Geometry: see drawing. Coordinates: mm, zero at the bounding-box minimum. Coordinates: 2 decimals unless noted, no trailing zeros. Write each loop counter-clockwise with the first axis right and the second up, starting at its lowest first coordinate (ties: lowest second). Pieces come first, ordered by that corner, then holes. Notation, with made-up numbers: (-16, -37.5) - (1, -37.5) arc R15 cw to (1, -21.5) - close; hole circle Ø9 at (15.5, -8.75). An arc over 180 degrees is marked (long way). One line per question, with ' | ' between items. Start each with the question number.
Q1. Cut plane A-A, the plane z = 26.5. Return loops of the section in (x, y), plus the area to 3 significant figures.
Q2. Contact query for flat-ended pins moving along their axis: P1, Ø1.5, axis at x = 23, y = 2, coming from the -Z side; P2, Ø1.5, axis at x = 23.5, y = 1.5, coming from the +Z side; P3, Ø0.9, axis at x = 22, y = 1.5, coming from the +Z side. Output: stop coordinate, or through.
Q3. Line query: line 1 (X direction, y = 1.3, z = 49); line 2 (Z direction, x = 62, y = 2.65) (1 decimal); line 3 (Z direction, x = 110, y = 2.05) (1 decimal). Output: solid intervals per line, ascending.
Q4. Cut plane B-B, the plane x = 128. Give the number of separate pieces and of enclosed holes in the cut face, plus the area to 3 significant figures.
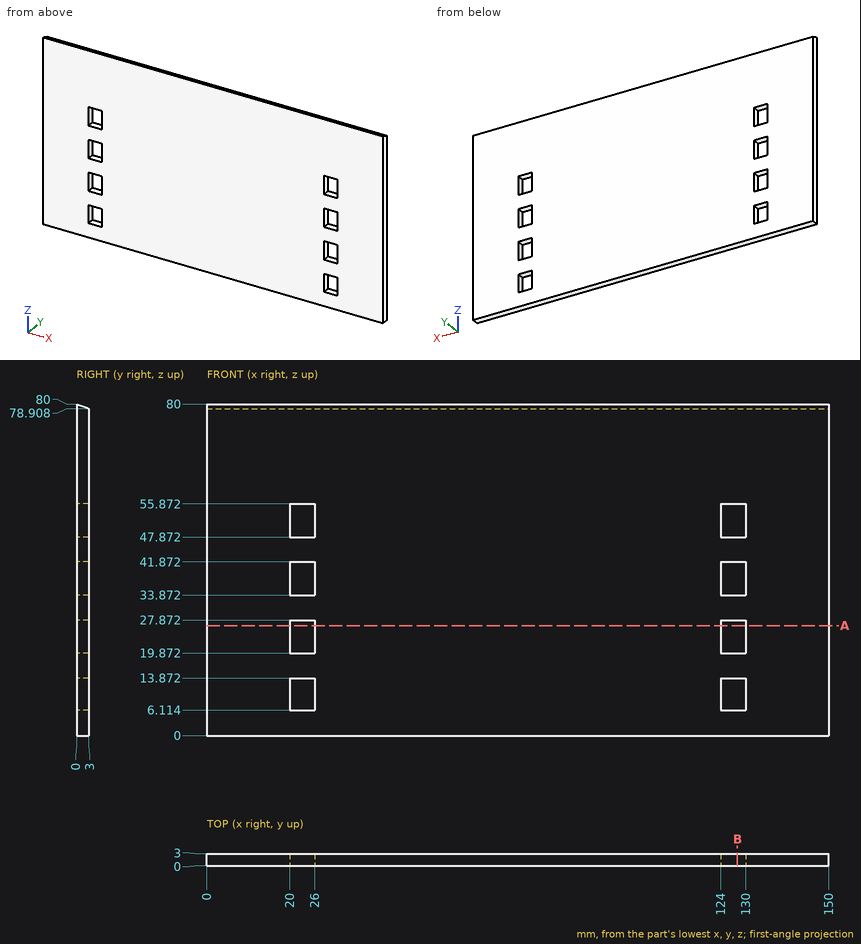
Reply:
1) outline: (0, 0) - (20, 0) - (20, 3) - (0, 3) - close; (26, 0) - (124, 0) - (124, 3) - (26, 3) - close; (130, 0) - (150, 0) - (150, 3) - (130, 3) - close | area: 414 mm^2
2) P1: stops at z = 0 | P2: stops at z = 79.73 | P3: stops at z = 79.62
3) line 1: x = 0 to 20, 26 to 124, 130 to 150 | line 2: z = 0 to 79 | line 3: z = 0 to 79.3
4) separate pieces: 5 | enclosed holes: 0 | area: 143 mm^2
